Could you check a few things on this model? Use its own coordinates, in mm. Give positions to 0.01 mm unless a question says otherwise; leave off trailing zeros. Write each loop counter-clockwise with the first axis right and the second up, starting at its lowest first coordinate (ties: lowest second). Pieces come first, ordered by that corner, then holes. Notation, with made-up numbers: M 18,-1.75 L 36,-1.75 A19 ccw 36,14.25 Z; hole C -25,-35 d10. An arc over 180 degrees is marked long. One line per item, written item: value.
```python
from build123d import *

# Parameters (mm, degrees)
SKETCH1_W           = 50.8
SKETCH1_H           = 3.175
BOSS_EXTRUDE1_DEPTH = 427.1518
SKETCH4_R           = 1.4224
CUT_EXTRUDE2_DEPTH  = 5.08
SKETCH5_W           = 12.58267919
SKETCH5_H           = 101.029760921
BOSS_EXTRUDE2_DEPTH = 3.175
SKETCH6_W           = 7.546607927
SKETCH6_H           = 108.671154153
SKETCH6_W_2         = 9.055929513
BOSS_EXTRUDE3_DEPTH = 3.175
SKETCH7_W           = 50.8
SKETCH7_H           = 16.51
BOSS_EXTRUDE4_DEPTH = 3.175
SKETCH8_W           = 50.8
SKETCH8_H           = 51.188017092
BOSS_EXTRUDE5_DEPTH = 3.175
SKETCH9_W           = 50.8
SKETCH9_H           = 70.169066632
BOSS_EXTRUDE6_DEPTH = 3.175
CUT_EXTRUDE3_DEPTH  = 428.918100655


with BuildPart() as part:
    # Sketch1 → Boss-Extrude1 (new body)
    with BuildSketch(Plane(origin=(0, 0, 0), x_dir=(1, 0, 0), z_dir=(0, 1, 0))):
        with Locations((0, 70.254548969)):
            Rectangle(SKETCH1_W, SKETCH1_H)
    extrude(amount=BOSS_EXTRUDE1_DEPTH)

    # Sketch4 → Cut-Extrude2 (cut)
    with BuildSketch(Plane.XY.offset(-68.667048969)):
        with Locations((-3.175, 376.3518)):
            Circle(SKETCH4_R)
        with Locations((-9.525, 376.3518)):
            Circle(SKETCH4_R)
        with Locations((-9.525, 370.0018)):
            Circle(SKETCH4_R)
        with Locations((-9.525, 363.6518)):
            Circle(SKETCH4_R)
        with Locations((-9.525, 357.3018)):
            Circle(SKETCH4_R)
        with Locations((-9.525, 350.9518)):
            Circle(SKETCH4_R)
        with Locations((-9.525, 344.6018)):
            Circle(SKETCH4_R)
        with Locations((-9.525, 338.2518)):
            Circle(SKETCH4_R)
        with Locations((-9.525, 331.9018)):
            Circle(SKETCH4_R)
        with Locations((-9.525, 325.5518)):
            Circle(SKETCH4_R)
        with Locations((-9.525, 319.2018)):
            Circle(SKETCH4_R)
        with Locations((-9.525, 312.8518)):
            Circle(SKETCH4_R)
        with Locations((-9.525, 306.5018)):
            Circle(SKETCH4_R)
        with Locations((-9.525, 300.1518)):
            Circle(SKETCH4_R)
        with Locations((-9.525, 293.8018)):
            Circle(SKETCH4_R)
        with Locations((-9.525, 287.4518)):
            Circle(SKETCH4_R)
        with Locations((-9.525, 281.1018)):
            Circle(SKETCH4_R)
        with Locations((-3.175, 370.0018)):
            Circle(SKETCH4_R)
        with Locations((-3.175, 363.6518)):
            Circle(SKETCH4_R)
        with Locations((-3.175, 357.3018)):
            Circle(SKETCH4_R)
        with Locations((-3.175, 350.9518)):
            Circle(SKETCH4_R)
        with Locations((-3.175, 344.6018)):
            Circle(SKETCH4_R)
        with Locations((-3.175, 338.2518)):
            Circle(SKETCH4_R)
        with Locations((-3.175, 331.9018)):
            Circle(SKETCH4_R)
        with Locations((-3.175, 325.5518)):
            Circle(SKETCH4_R)
        with Locations((-3.175, 319.2018)):
            Circle(SKETCH4_R)
        with Locations((-3.175, 312.8518)):
            Circle(SKETCH4_R)
        with Locations((-3.175, 306.5018)):
            Circle(SKETCH4_R)
        with Locations((-3.175, 300.1518)):
            Circle(SKETCH4_R)
        with Locations((-3.175, 293.8018)):
            Circle(SKETCH4_R)
        with Locations((-3.175, 287.4518)):
            Circle(SKETCH4_R)
        with Locations((-3.175, 281.1018)):
            Circle(SKETCH4_R)
        with Locations((3.175, 281.1018)):
            Circle(SKETCH4_R)
        with Locations((3.175, 287.4518)):
            Circle(SKETCH4_R)
        with Locations((3.175, 293.8018)):
            Circle(SKETCH4_R)
        with Locations((3.175, 300.1518)):
            Circle(SKETCH4_R)
        with Locations((3.175, 306.5018)):
            Circle(SKETCH4_R)
        with Locations((3.175, 312.8518)):
            Circle(SKETCH4_R)
        with Locations((3.175, 319.2018)):
            Circle(SKETCH4_R)
        with Locations((3.175, 325.5518)):
            Circle(SKETCH4_R)
        with Locations((3.175, 331.9018)):
            Circle(SKETCH4_R)
        with Locations((3.175, 338.2518)):
            Circle(SKETCH4_R)
        with Locations((3.175, 344.6018)):
            Circle(SKETCH4_R)
        with Locations((3.175, 350.9518)):
            Circle(SKETCH4_R)
        with Locations((3.175, 357.3018)):
            Circle(SKETCH4_R)
        with Locations((3.175, 363.6518)):
            Circle(SKETCH4_R)
        with Locations((3.175, 370.0018)):
            Circle(SKETCH4_R)
        with Locations((9.525, 281.1018)):
            Circle(SKETCH4_R)
        with Locations((9.525, 287.4518)):
            Circle(SKETCH4_R)
        with Locations((9.525, 293.8018)):
            Circle(SKETCH4_R)
        with Locations((9.525, 300.1518)):
            Circle(SKETCH4_R)
        with Locations((9.525, 306.5018)):
            Circle(SKETCH4_R)
        with Locations((9.525, 312.8518)):
            Circle(SKETCH4_R)
        with Locations((9.525, 319.2018)):
            Circle(SKETCH4_R)
        with Locations((9.525, 325.5518)):
            Circle(SKETCH4_R)
        with Locations((9.525, 331.9018)):
            Circle(SKETCH4_R)
        with Locations((9.525, 338.2518)):
            Circle(SKETCH4_R)
        with Locations((9.525, 344.6018)):
            Circle(SKETCH4_R)
        with Locations((9.525, 350.9518)):
            Circle(SKETCH4_R)
        with Locations((9.525, 357.3018)):
            Circle(SKETCH4_R)
        with Locations((9.525, 363.6518)):
            Circle(SKETCH4_R)
        with Locations((9.525, 370.0018)):
            Circle(SKETCH4_R)
        with Locations((9.525, 376.3518)):
            Circle(SKETCH4_R)
        with Locations((3.175, 376.3518)):
            Circle(SKETCH4_R)
        with Locations((-9.525, 382.7018)):
            Circle(SKETCH4_R)
        with Locations((9.525, 382.7018)):
            Circle(SKETCH4_R)
        with Locations((-9.525, 389.0518)):
            Circle(SKETCH4_R)
        with Locations((9.525, 389.0518)):
            Circle(SKETCH4_R)
        with Locations((-9.525, 395.4018)):
            Circle(SKETCH4_R)
        with Locations((9.525, 395.4018)):
            Circle(SKETCH4_R)
        with Locations((-9.525, 401.7518)):
            Circle(SKETCH4_R)
        with Locations((9.525, 401.7518)):
            Circle(SKETCH4_R)
        with Locations((-9.525, 408.1018)):
            Circle(SKETCH4_R)
        with Locations((9.525, 408.1018)):
            Circle(SKETCH4_R)
        with Locations((-9.525, 414.4518)):
            Circle(SKETCH4_R)
        with Locations((9.525, 414.4518)):
            Circle(SKETCH4_R)
    cut_extrude2 = extrude(amount=-CUT_EXTRUDE2_DEPTH, mode=Mode.SUBTRACT)

    # Sketch5 → Boss-Extrude2 (add)
    with BuildSketch(Plane.XY.offset(-68.667048969)):
        with Locations((-0.175223229, 328.362881378)):
            Rectangle(SKETCH5_W, SKETCH5_H)
    boss_extrude2 = extrude(amount=-BOSS_EXTRUDE2_DEPTH)

    # Sketch6 → Boss-Extrude3 (add)
    with BuildSketch(Plane.XY.offset(-68.667048969)):
        with Locations((-16.484092579, 326.705642943)):
            Rectangle(SKETCH6_W, SKETCH6_H)
        with Locations((16.9725359, 326.705642943)):
            Rectangle(SKETCH6_W_2, SKETCH6_H)
    boss_extrude3 = extrude(amount=-BOSS_EXTRUDE3_DEPTH)

    # Sketch7 → Boss-Extrude4 (add)
    with BuildSketch(Plane.XY.offset(-68.667048969)):
        with Locations((0, 418.8968)):
            Rectangle(SKETCH7_W, SKETCH7_H)
    boss_extrude4 = extrude(amount=-BOSS_EXTRUDE4_DEPTH)

    # Sketch8 → Boss-Extrude5 (add)
    with BuildSketch(Plane.XY.offset(-68.667048969)):
        with Locations((0, 379.332910144)):
            Rectangle(SKETCH8_W, SKETCH8_H)
    boss_extrude5 = extrude(amount=-BOSS_EXTRUDE5_DEPTH)

    # Sketch9 → Boss-Extrude6 (add)
    with BuildSketch(Plane.XY.offset(-68.667048969)):
        with Locations((0, 312.515447534)):
            Rectangle(SKETCH9_W, SKETCH9_H)
    boss_extrude6 = extrude(amount=-BOSS_EXTRUDE6_DEPTH)

    # Mirror1: Cut-Extrude2, Boss-Extrude2, Boss-Extrude3, Boss-Extrude4, Boss-Extrude5, Boss-Extrude6 across plane
    add(cut_extrude2.mirror(Plane.ZX.offset(213.5759)), mode=Mode.SUBTRACT)
    add(boss_extrude2.mirror(Plane.ZX.offset(213.5759)))
    add(boss_extrude3.mirror(Plane.ZX.offset(213.5759)))
    add(boss_extrude4.mirror(Plane.ZX.offset(213.5759)))
    add(boss_extrude5.mirror(Plane.ZX.offset(213.5759)))
    add(boss_extrude6.mirror(Plane.ZX.offset(213.5759)))

    # Sketch11 → Cut-Extrude3 (cut, through all)
    with BuildSketch(Plane.XY.offset(-68.667048969)):
        with BuildLine():
            Line((9.292893219, 105.9942), (-9.292893219, 105.9942))
            ThreePointArc((-9.292893219, 105.9942), (-10, 105.9942), (-10, 106.701306781))
            Line((-10, 106.701306781), (-10, 108.462093219))
            ThreePointArc((-10, 108.462093219), (-10, 109.1692), (-9.292893219, 109.1692))
            Line((-9.292893219, 109.1692), (9.292893219, 109.1692))
            ThreePointArc((9.292893219, 109.1692), (10, 109.1692), (10, 108.462093219))
            Line((10, 108.462093219), (10, 106.701306781))
            ThreePointArc((10, 106.701306781), (10, 105.9942), (9.292893219, 105.9942))
        make_face()
        with BuildLine():
            Line((9.292893219, 0), (-9.292893219, 0))
            ThreePointArc((-9.292893219, 0), (-10, 0), (-10, 0.707106781))
            Line((-10, 0.707106781), (-10, 2.467893219))
            ThreePointArc((-10, 2.467893219), (-10, 3.175), (-9.292893219, 3.175))
            Line((-9.292893219, 3.175), (9.292893219, 3.175))
            ThreePointArc((9.292893219, 3.175), (10, 3.175), (10, 2.467893219))
            Line((10, 2.467893219), (10, 0.707106781))
            ThreePointArc((10, 0.707106781), (10, 0), (9.292893219, 0))
        make_face()
        with BuildLine():
            Line((9.292893219, 211.9884), (-9.292893219, 211.9884))
            ThreePointArc((-9.292893219, 211.9884), (-10, 211.9884), (-10, 212.695506781))
            Line((-10, 212.695506781), (-10, 214.456293219))
            ThreePointArc((-10, 214.456293219), (-10, 215.1634), (-9.292893219, 215.1634))
            Line((-9.292893219, 215.1634), (9.292893219, 215.1634))
            ThreePointArc((9.292893219, 215.1634), (10, 215.1634), (10, 214.456293219))
            Line((10, 214.456293219), (10, 212.695506781))
            ThreePointArc((10, 212.695506781), (10, 211.9884), (9.292893219, 211.9884))
        make_face()
    cut_extrude3 = extrude(amount=-CUT_EXTRUDE3_DEPTH, mode=Mode.SUBTRACT)

    # Mirror2: Cut-Extrude3 across plane
    add(cut_extrude3.mirror(Plane(origin=(0, 213.5759, 0), x_dir=(0, 0, 1), z_dir=(0, -1, 0))), mode=Mode.SUBTRACT)


solid = part.part
```
1) Please list where these lines run through material, in increasing order: L1, parallel to Y at x = 2.5, z = -68.8 (3 decimals); L2, parallel to X at y = 19.05, z = -70.65. Write a range as from..to.
Outcome:
L1: y = 3.175..105.994, 109.169..211.988, 215.163..317.983, 321.158..423.977
L2: x = -25.4..-10.95, -8.1..8.1, 10.95..25.4
2) If we section it at B-B, the plane z = -71.1: Give the number of separate pieces and of enclosed holes in the cut face, then the cut area to 3 significant figures.
Outcome:
separate pieces: 1
enclosed holes: 11
area: 21,300 mm^2
3) I'm going to push flat-ended pins straight in: pin 1 (3.5 mm diameter, centred on x = 9.52, y = 350.95, fed in from -Z); pin 2 (1.7 mm diameter, centred on x = -9.52, y = 408.1, fed in from +Z); pin 3 (1 mm diameter, centred on x = -2, z = -71, fed in from -Y) (3 decimals); pin 4 (1 mm diameter, centred on x = 3, z = -70, fed in from +Y). Where does each tip first touch, or does it pass through?
Outcome:
pin 1: stops at z = -71.84
pin 2: passes through
pin 3: stops at y = 3.175
pin 4: stops at y = 423.98
4) If we section it at A-A, the plane x = -1: Write out the boundary of the cut face in (y, z) (3 decimals), then the cut area to 3 significant figures.
Outcome:
outline: M 3.175,-71.842 L 105.994,-71.842 L 105.994,-68.667 L 3.175,-68.667 Z; M 109.169,-71.842 L 211.988,-71.842 L 211.988,-68.667 L 109.169,-68.667 Z; M 215.163,-71.842 L 317.983,-71.842 L 317.983,-68.667 L 215.163,-68.667 Z; M 321.158,-71.842 L 423.977,-71.842 L 423.977,-68.667 L 321.158,-68.667 Z
area: 1,310 mm^2
